```python
from build123d import *

# Parameters (mm, degrees)
SKETCH1_R           = 3.2385
BOSS_EXTRUDE1_DEPTH = 8.255
SKETCH3_W           = 3.302
SKETCH3_H           = 38.1
SKETCH3_W_2         = 38.1
SKETCH3_H_2         = 3.302
BOSS_EXTRUDE3_DEPTH = 25.4
SKETCH5_R           = 2.159
CUT_EXTRUDE1_DEPTH  = 204.327
SKETCH6_W           = 12.7
SKETCH6_H           = 3.302
BOSS_EXTRUDE5_DEPTH = 25.4
CUT_EXTRUDE2_DEPTH  = 25.4
SKETCH8_W           = 3.302
SKETCH8_H           = 12.7
BOSS_EXTRUDE6_DEPTH = 25.4
CUT_EXTRUDE3_DEPTH  = 25.4
FILLET1_R           = 2.54


with BuildPart() as part:
    # Sketch1 → Boss-Extrude1 (new body)
    with BuildSketch(Plane(origin=(0, 0, 0), x_dir=(1, 0, 0), z_dir=(0, 1, 0))):
        with BuildLine():
            Line((-1.651, 166.628963684), (-1.651, 14.89477744))
            ThreePointArc((-1.651, 14.89477744), (-10.596702223, -10.596702223), (14.89477744, -1.651))
            Line((14.89477744, -1.651), (166.628963684, -1.651))
            Line((166.628963684, -1.651), (180.975, -19.05))
            Line((180.975, -19.05), (180.975, -15.057345133))
            Line((180.975, -15.057345133), (169.921036316, -1.651))
            Line((169.921036316, -1.651), (180.975, -1.651))
            Line((180.975, -1.651), (180.975, 1.651))
            Line((180.975, 1.651), (169.921036316, 1.651))
            Line((169.921036316, 1.651), (180.975, 15.057345133))
            Line((180.975, 15.057345133), (180.975, 19.05))
            Line((180.975, 19.05), (166.628963684, 1.651))
            Line((166.628963684, 1.651), (144.671051224, 1.651))
            Line((144.671051224, 1.651), (1.651, 144.671051224))
            Line((1.651, 144.671051224), (1.651, 166.628963684))
            Line((1.651, 166.628963684), (19.05, 180.975))
            Line((19.05, 180.975), (15.057345133, 180.975))
            Line((15.057345133, 180.975), (1.651, 169.921036316))
            Line((1.651, 169.921036316), (1.651, 180.975))
            Line((1.651, 180.975), (-1.651, 180.975))
            Line((-1.651, 180.975), (-1.651, 169.921036316))
            Line((-1.651, 169.921036316), (-15.057345133, 180.975))
            Line((-15.057345133, 180.975), (-19.05, 180.975))
            Line((-19.05, 180.975), (-1.651, 166.628963684))
        make_face()
        with BuildLine():
            Line((-9.686234559, -5.271576621), (-7.236078848, -3.458556767))
            ThreePointArc((-7.236078848, -3.458556767), (-5.104491065, -3.777124696), (-5.423058993, -5.908712478))
            Line((-5.423058993, -5.908712478), (-7.873214705, -7.721732332))
            ThreePointArc((-7.873214705, -7.721732332), (-10.004802487, -7.403164404), (-9.686234559, -5.271576621))
        make_face(mode=Mode.SUBTRACT)
        Circle(SKETCH1_R, mode=Mode.SUBTRACT)
        with BuildLine():
            ThreePointArc((7.236078848, 3.458556767), (5.104491065, 3.777124696), (5.423058993, 5.908712478))
            Line((5.423058993, 5.908712478), (7.873214705, 7.721732332))
            ThreePointArc((7.873214705, 7.721732332), (10.004802487, 7.403164404), (9.686234559, 5.271576621))
            Line((9.686234559, 5.271576621), (7.236078848, 3.458556767))
        make_face(mode=Mode.SUBTRACT)
        with BuildLine():
            Line((77.202140867, 1.651), (14.89477744, 1.651))
            ThreePointArc((14.89477744, 1.651), (10.596702223, 10.596702223), (1.651, 14.89477744))
            Line((1.651, 14.89477744), (1.651, 77.202140867))
            Line((1.651, 77.202140867), (65.527807909, 77.202140867))
            Line((65.527807909, 77.202140867), (77.202140867, 65.527807909))
            Line((77.202140867, 65.527807909), (77.202140867, 1.651))
        make_face(mode=Mode.SUBTRACT)
        Polygon((141.078948776, 1.651), (81.012140867, 1.651), (81.012140867, 61.717807909), align=None, mode=Mode.SUBTRACT)
        Polygon((1.651, 81.012140867), (1.651, 141.078948776), (61.717807909, 81.012140867), align=None, mode=Mode.SUBTRACT)
    extrude(amount=BOSS_EXTRUDE1_DEPTH)

    # Sketch3 → Boss-Extrude3 (add)
    with BuildSketch(Plane(origin=(0, 0, 0), x_dir=(1, 0, 0), z_dir=(0, 1, 0))):
        with Locations((182.626, 0)):
            Rectangle(SKETCH3_W, SKETCH3_H)
        with Locations((0, 182.626)):
            Rectangle(SKETCH3_W_2, SKETCH3_H_2)
    extrude(amount=BOSS_EXTRUDE3_DEPTH)

    # Sketch5 → Cut-Extrude1 (cut, through all)
    with BuildSketch(Plane(origin=(184.277, 0, 0), x_dir=(0, 0, -1), z_dir=(1, 0, 0))):
        with Locations((-9.525, 12.7)):
            Circle(SKETCH5_R)
        with Locations((9.525, 12.7)):
            Circle(SKETCH5_R)
    cut_extrude1 = extrude(amount=-CUT_EXTRUDE1_DEPTH, mode=Mode.SUBTRACT)

    # Mirror1: Cut-Extrude1 across plane
    add(cut_extrude1.mirror(Plane(origin=(0, 0, 0), x_dir=(-0.707106781, 0, 0.707106781), z_dir=(0.707106781, 0, 0.707106781))), mode=Mode.SUBTRACT)

    # Sketch6 → Boss-Extrude5 (add)
    with BuildSketch(Plane(origin=(0, 0, 0), x_dir=(1, 0, 0), z_dir=(0, 1, 0))):
        with Locations((174.625, 0)):
            Rectangle(SKETCH6_W, SKETCH6_H)
    extrude(amount=BOSS_EXTRUDE5_DEPTH)

    # Sketch7 → Cut-Extrude2 (cut)
    with BuildSketch(Plane(origin=(0, 0, -1.651), x_dir=(-1, 0, 0), z_dir=(0, 0, -1))):
        Polygon((-180.975, 25.4), (-168.275, 8.255), (-168.275, 25.4), align=None)
    extrude(amount=-CUT_EXTRUDE2_DEPTH, mode=Mode.SUBTRACT)

    # Sketch8 → Boss-Extrude6 (add)
    with BuildSketch(Plane(origin=(0, 0, 0), x_dir=(1, 0, 0), z_dir=(0, 1, 0))):
        with Locations((0, 174.625)):
            Rectangle(SKETCH8_W, SKETCH8_H)
    extrude(amount=BOSS_EXTRUDE6_DEPTH)

    # Sketch9 → Cut-Extrude3 (cut)
    with BuildSketch(Plane(origin=(1.651, 0, 0), x_dir=(0, 0, -1), z_dir=(1, 0, 0))):
        Polygon((180.975, 25.4), (168.275, 8.255), (168.275, 25.4), align=None)
    extrude(amount=-CUT_EXTRUDE3_DEPTH, mode=Mode.SUBTRACT)

    # Fillet1
    fillet1_edges = [part.edges().sort_by_distance(p)[0] for p in [
        (-1.651, 4.1275, -166.628963684),
        (-1.651, 4.1275, -169.921036316),
        (-1.651, 12.7, -180.975),
        (1.651, 12.7, -180.975),
        (1.651, 4.1275, -169.921036316),
        (1.651, 4.1275, -166.628963684),
        (1.651, 4.1275, -144.671051224),
        (144.671051224, 4.1275, -1.651),
        (166.628963684, 4.1275, -1.651),
        (169.921036316, 4.1275, -1.651),
        (180.975, 12.7, -1.651),
        (180.975, 12.7, 1.651),
        (169.921036316, 4.1275, 1.651),
        (166.628963684, 4.1275, 1.651),
        (14.89477744, 4.1275, 1.651),
        (-1.651, 4.1275, -14.89477744),
        (61.717807909, 4.1275, -81.012140867),
        (1.651, 4.1275, -141.078948776),
        (1.651, 4.1275, -81.012140867),
        (77.202140867, 4.1275, -1.651),
        (77.202140867, 4.1275, -65.527807909),
        (65.527807909, 4.1275, -77.202140867),
        (1.651, 4.1275, -77.202140867),
        (1.651, 4.1275, -14.89477744),
        (14.89477744, 4.1275, -1.651),
        (141.078948776, 4.1275, -1.651),
        (81.012140867, 4.1275, -61.717807909),
        (81.012140867, 4.1275, -1.651),
    ]]
    fillet(fillet1_edges, radius=FILLET1_R)


solid = part.part
```
The model under review builds one solid part; all positions refer to its coordinate system, in mm. A direction names the side the tool comes from. Round coordinates to 2 decimals unless told otherwise and drop trailing zeros. Order: outer loops, then holes, each group sorted by start corner. A loop starts at its lowest first (then second) coordinate and runs counter-clockwise, first axis right, second up. Notation, with made-up numbers: (11.5, 77.25) -> (60.5, 77.25) arc R24 ccw to (60.5, 95.25) -> close; hole circle Ø11 at (59.25, -38). An arc over 180 degrees is marked (long way). One line per item, written item: value. Start each with the question number.
Q1. Wall thickness on line 1 (X direction, y = 12.7, z = -183.05); line 2 (X direction, y = 5.75, z = -2); line 3 (X direction, y = 3.25, z = -111.5): over which ranges is each line inside the solid? List them lowest first.
Q2. Take a section at B-B (z = -108.5). Write out the cut boundary in (x, y) (3 decimals), and give its area (3 significant figures).
Q3. Take a section at A-A (x = 44.5). Write out the cut boundary in (y, z) (3 decimals).
Q4. Clearance check with flat-ended pins moving along their axes: pin 1 Ø5 at (y, z) = (13.5, -175.5) entering from -X; pin 2 Ø4 at (y, z) = (6, -159.5) entering from +X; pin 3 Ø6.5 at (x, y) = (37, 3.5) entering from -Z; pin 4 Ø4 at (x, y) = (62.5, 11) entering from +Z. State where each tip first meets the part, or that it passes through.
Q5. Mouldability with a two-part tool opening along X and no side actions: class faces 1 (the face through (3.26, 4.19, -137.31)), 2 (the face through (10.7, 4.07, -174.09)), 3 (the face through (60, 0, -83)) as released by +X, released by -X, zero draft, split by the parting line, or undercut.
Q6. Machinability: for faces 4 (the face through (176, 11, 1.651)), 5 (the face through (90, 4, 1.651)), 6 (the face through (-1.651, 4, -92)), 7 (the face through (31.32, 4.07, -111.41)), 8 (the face through (175.125, 17.503, -0.02)), which of the approach directions +Z, -Z, +X, -X, +Y, -Y give a long, thin tool a straight path to every point of the face, cutting with its end or side? Answer none if there is none.
Q7. Take a section at C-C (y = 5.75). Count the separate pieces of the cut face and the enclosed holes in it, and give its area (3 significant figures).
Q8. Take a section at D-D (z = -47). Write out the cut boundary in (x, y) (3 decimals).
Reported:
1. line 1: x = -19.05 to -11.68, -7.37 to 7.37, 11.68 to 19.05
1. line 2: x = -14.85 to -2.55, 2.55 to 15.73, 75.95 to 82.27, 136.23 to 144.44, 166.72 to 174.02, 179.72 to 184.28
1. line 3: x = -1.65 to 1.65, 31.23 to 34.82
2. outline: (-1.651, 0) -> (1.651, 0) -> (1.651, 8.255) -> (-1.651, 8.255) -> close; (34.23, 0) -> (37.822, 0) -> (37.822, 8.255) -> (34.23, 8.255) -> close
2. area: 56.9 mm2
3. outline: (0, -101.822) -> (8.255, -101.822) -> (8.255, -98.23) -> (0, -98.23) -> close; (0, -81.012) -> (8.255, -81.012) -> (8.255, -77.202) -> (0, -77.202) -> close; (0, -1.651) -> (8.255, -1.651) -> (8.255, 1.651) -> (0, 1.651) -> close
4. pin 1: stops at x = -1.65
4. pin 2: stops at x = 1.65
4. pin 3: stops at z = -112.57
4. pin 4: passes through
5. face 1: undercut
5. face 2: released by +X
5. face 3: zero draft
6. face 4: +Y
6. face 5: +Z, +Y, -Y
6. face 6: -X, +Y, -Y
6. face 7: +Y, -Y
6. face 8: +Z, -Z, -X, +Y
7. separate pieces: 1
7. enclosed holes: 10
7. area: 3,240 mm2
8. outline: (-1.651, 0) -> (1.651, 0) -> (1.651, 8.255) -> (-1.651, 8.255) -> close; (77.202, 0) -> (81.012, 0) -> (81.012, 8.255) -> (77.202, 8.255) -> close; (95.73, 0) -> (99.322, 0) -> (99.322, 8.255) -> (95.73, 8.255) -> close
